Check sheet for the modelled part. Datum: model origin and axes. Units: mm. A direction names the side the tool comes from. Give positions to 0.01 mm unless a question says otherwise; leave off trailing zeros. Order: outer loops, then holes, each group sorted by start corner. A loop starts at its lowest first (then second) coordinate and runs counter-clockwise, first axis right, second up.
```python
from build123d import *

# Parameters (mm, degrees)
F1_DEPTH    = 50
F2_DEPTH    = 3
F3_T1_DEPTH = 28
F3_T3_DEPTH = 33.9128784748
F4_DEPTH    = 120
F5_T1_DEPTH = 102.6362149123
F5_T3_DEPTH = 102.6362149123
F6_R        = 11
F7_DEPTH    = 4
F8_R        = 7
F9_DEPTH    = 17
F10_R       = 5


# Not quite as in the source:
# - a fillet or chamfer that OpenCascade refuses, or shapes differently, is made with other operations: its cross-section is extruded or revolved along the edge and cut away or added


with BuildPart() as f1:
    # F0 (on Front) → F1 (new body)
    with BuildSketch(Plane.XZ):
        Polygon((26.5539305929, 3.625), (-26.5539305929, 3.625), (-19.7357487747, -6.375), (19.7357487747, -6.375), align=None)
    extrude(amount=F1_DEPTH)

    # F0 (on Front) → F2 (join)
    with BuildSketch(Plane.XZ):
        Polygon((20, -6.875), (-20, -6.875), (-27.1590909091, 3.625), (-27.5, 3.625), (-28.5, 3.625), (-28.5, -7.375), (28.5, -7.375), (28.5, 3.625), (27.5, 3.625), (27.1590909091, 3.625), align=None)
        Polygon((26.5539305929, 3.625), (-26.5539305929, 3.625), (-19.7357487747, -6.375), (19.7357487747, -6.375), align=None)
        Polygon((-27.1590909091, 3.625), (-20, -6.875), (20, -6.875), (27.1590909091, 3.625), (26.5539305929, 3.625), (19.7357487747, -6.375), (-19.7357487747, -6.375), (-26.5539305929, 3.625), align=None)
    extrude(amount=F2_DEPTH)

    # F3: fillet of radius 5 on 4 edges, made by hand

    # F3_s2 → F3_t1 (cut)
    with BuildSketch(Plane.XZ.offset(-12.5)):
        with BuildLine():
            ThreePointArc((28.5, -2.375), (27.0355339059, -5.9105339059), (23.5, -7.375))
            Line((23.5, -7.375), (28.5, -7.375))
            Line((28.5, -7.375), (28.5, -2.375))
        make_face()
        with BuildLine():
            ThreePointArc((-23.5, -7.375), (-27.0355339059, -5.9105339059), (-28.5, -2.375))
            Line((-28.5, -2.375), (-28.5, -7.375))
            Line((-28.5, -7.375), (-23.5, -7.375))
        make_face()
    extrude(amount=F3_T1_DEPTH, mode=Mode.SUBTRACT)

    # F3_s4 → F3_t3 (cut)
    with BuildSketch(Plane.XY.offset(-18.8314392374)):
        with BuildLine():
            ThreePointArc((23.917424305, 0), (26.6560370926, -0.8166998673), (28.5, -3))
            Line((28.5, -3), (28.5, 0))
            Line((28.5, 0), (23.917424305, 0))
        make_face()
        with BuildLine():
            ThreePointArc((-23.917424305, 0), (-26.6560370926, -0.8166998673), (-28.5, -3))
            Line((-28.5, -3), (-28.5, 0))
            Line((-28.5, 0), (-23.917424305, 0))
        make_face()
    extrude(amount=F3_T3_DEPTH, mode=Mode.SUBTRACT)

    # F0 (on Front) → F4 (join)
    with BuildSketch(Plane.XZ):
        Polygon((26.5539305929, 3.625), (-26.5539305929, 3.625), (-19.7357487747, -6.375), (19.7357487747, -6.375), align=None)
    extrude(amount=-F4_DEPTH)

    # F5: fillet of radius 18.1066017178 on 2 edges, made by hand

    # F5_s2 → F5_t1 (cut)
    with BuildSketch(Plane(origin=(-22.2043882639, 0, -32.5664361204), x_dir=(0, 1, 0), z_dir=(0.5633368246, 0, 0.8262273428))):
        with BuildLine():
            ThreePointArc((101.8933982822, -19.8974875256), (114.6966991411, -14.5941866667), (120, -1.7908858078))
            Line((120, -1.7908858078), (120, -19.8974875256))
            Line((120, -19.8974875256), (101.8933982822, -19.8974875256))
        make_face()
    extrude(amount=F5_T1_DEPTH, mode=Mode.SUBTRACT)

    # F5_s4 → F5_t3 (cut)
    with BuildSketch(Plane(origin=(-35.614371138, 0, 52.2344110024), x_dir=(0, 1, 0), z_dir=(0.5633368246, 0, -0.8262273428))):
        with BuildLine():
            ThreePointArc((101.8933982822, -19.8974875256), (114.6966991411, -14.5941866667), (120, -1.7908858078))
            Line((120, -1.7908858078), (120, -19.8974875256))
            Line((120, -19.8974875256), (101.8933982822, -19.8974875256))
        make_face()
    extrude(amount=F5_T3_DEPTH, mode=Mode.SUBTRACT)

    # F6 (on face) → F7 (join)
    with BuildSketch(Plane(origin=(0, 0, -6.375), x_dir=(1, 0, 0), z_dir=(0, 0, -1))):
        with Locations((0, -105.7220622897)):
            Circle(F6_R)
    extrude(amount=F7_DEPTH)

    # F8 (on face) → F9 (join)
    with BuildSketch(Plane(origin=(0, 0, -10.375), x_dir=(1, 0, 0), z_dir=(0, 0, -1))):
        with Locations((0, -105.7220622897)):
            Circle(F8_R)
    extrude(amount=F9_DEPTH)

    # F10
    f10_edges = [f1.edges().sort_by_distance(p)[0] for p in [
        (23.14484, -50, -1.375),
        (-23.14484, -50, -1.375),
    ]]
    fillet(f10_edges, radius=F10_R)


solid = f1.part
```
(1) Material ranges on L1, parallel to Z at x = -13.5, y = 111 (3 decimals); L2, parallel to Y at x = -15, z = -6.5; L3, parallel to Y at x = -25.5, z = -1, recorded low to high.
Response values:
L1: z = -6.375 to 3.625
L2: y = -3 to 0
L3: y = -3 to -0.26
(2) Gauge pin test, flat ends, axial feed: pin 1 Ø2 at (x, z) = (-25.5, 1) entering from -Y; pin 2 Ø1.5 at (y, z) = (10, -1) entering from -X; pin 3 Ø1.5 at (y, z) = (3.5, -9) entering from -X; pin 4 Ø4 at (y, z) = (75.5, -3.5) entering from +X. Record the tip position at first contact, or that the pin passes through.
Response values:
pin 1: stops at y = -46.94
pin 2: stops at x = -23.91
pin 3: passes through
pin 4: stops at x = 23.06
(3) Set-up check for faces 4 (the face through (23.097, 50.233, -1.445)), 5 (the face through (23.1, -23.71, -1.44)), 6 (the face through (-23.19, 50.23, -1.31)), 7 (the face through (0, -3, -7)): record each of +Z, -Z, +X, -X, +Y, -Y from which the full face is reachable in a straight line by a thin tool's end or side.
Response values:
face 4: -Z, +X, +Y
face 5: -Z, +X, -Y
face 6: -Z, -X, +Y
face 7: -Z, -Y
(4) Cross-section at C-C on y = -31. Enter the section's corners in (x, z) (3 decimals).
Response values:
outline: (-26.554, 3.625) - (-19.736, -6.375) - (19.736, -6.375) - (26.554, 3.625) - close
(5) Cross-section at B-B on z = -19. Enter the section's corners in (x, y).
Response values:
outline: circle Ø14 at (0, 105.72)
(6) Cross-section at A-A on y = 97. Enter the section's corners in (x, z) (3 decimals).
Response values:
outline: (-26.554, 3.625) - (-19.736, -6.375) - (-6.703, -6.375) - (-6.703, -10.375) - (6.703, -10.375) - (6.703, -6.375) - (19.736, -6.375) - (26.554, 3.625) - close
(7) Release check for a two-part mould opening along Y. For faces 1 (the face through (-20.881, -48.574, -2.026)), 2 (the face through (-17.29, 114.56, -0.79)), 3 (the face through (0, 46, -6.375)) record: released by +Y, released by -Y, zero draft, split by the parting line, or undercut.
Response values:
face 1: released by -Y
face 2: released by +Y
face 3: undercut
